Could you check a few things on this drawing? It's one solid part, dimensions in mm from its lowest x, y, z. A direction names the side the tool comes from. Give positions to 0.01 mm unless a question says otherwise; leave off trailing zeros. Order: outer loops, then holes, each group sorted by start corner. A loop starts at its lowest first (then second) coordinate and runs counter-clockwise, first axis right, second up. Notation, with made-up numbers: (-11.75, 75) - (29.25, 75) arc R15 cw to (29.25, 89) - close; hole circle Ø10 at (-12.5, 29.5). An arc over 180 degrees is marked (long way). Put each result on its own line as item: value.
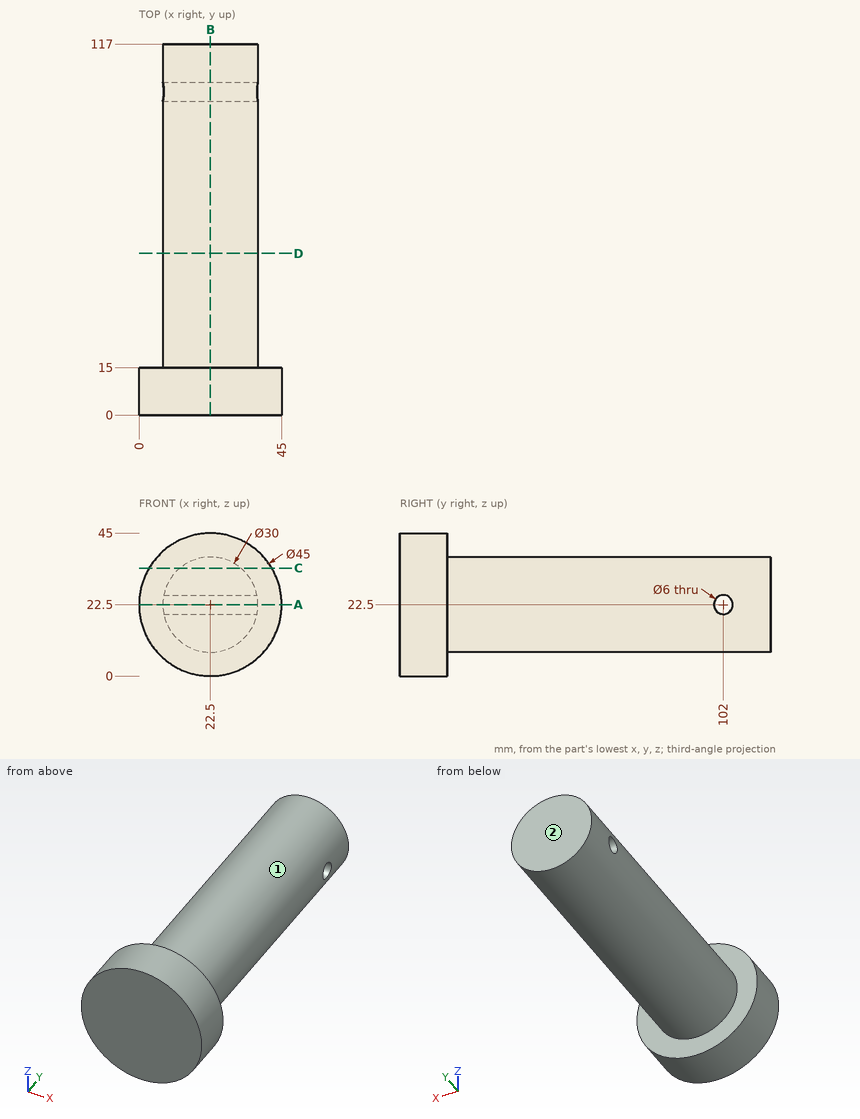
1) Suppose I cut it at D-D, the plane y = 51. List the corners of the cut face in (x, z) for me, and give its area (3 significant figures).
Filled in:
outline: circle Ø30 at (22.5, 22.5)
area: 707 mm^2
2) Which directions (+Z, -Z, +X, -X, +Y, -Y) give clear straight access to the entire face, cutting with the end or side of a thin tool? Please do the marked faces 1 and 2.
Filled in:
face 1: +Y
face 2: +Z, -Z, +X, -X, +Y
3) Suppose I cut it at B-B, the plane x = 22.5. List the corners of the cut face in (y, z) for me.
Filled in:
outline: (0, 0) - (15, 0) - (15, 7.5) - (117, 7.5) - (117, 37.5) - (15, 37.5) - (15, 45) - (0, 45) - close; hole circle Ø6 at (102, 22.5)
4) I'm going to push flat-ended pins straight in: pin 1 (8 mm diameter, centred on x = 9, y = 84.5, fed in from -Z); pin 2 (1.5 mm diameter, centred on y = 17, z = 28.5, fed in from +X); pin 3 (5 mm diameter, centred on y = 35.5, z = 37.5, fed in from +X). Where does each tip first touch, or does it pass through?
Filled in:
pin 1: stops at z = 10.89
pin 2: stops at x = 36.55
pin 3: stops at x = 30.79
5) Suppose I cut it at C-C, the plane z = 34. List the corners of the cut face in (x, y) for me, and give its area (3 significant figures).
Filled in:
outline: (3.16, 0) - (41.84, 0) - (41.84, 15) - (32.13, 15) - (32.13, 117) - (12.87, 117) - (12.87, 15) - (3.16, 15) - close
area: 2,540 mm^2
6) Suppose I cut it at A-A, the plane z = 22.5. List the corners of the cut face in (x, y) for me, and give its area (4 significant figures).
Filled in:
outline: (0, 0) - (45, 0) - (45, 15) - (37.5, 15) - (37.5, 99) - (7.5, 99) - (7.5, 15) - (0, 15) - close; (7.5, 105) - (37.5, 105) - (37.5, 117) - (7.5, 117) - close
area: 3,555 mm^2
7) If I drill on line 1 (Y direction, x = 26, z = 22.5); line 2 (Y direction, x = 19, z = 23.5); line 3 (Z direction, x = 29, y = 102), over which ranges is the centre line in solid material (lowest first)? Write a range as [from, to].
Filled in:
line 1: y = [0, 99], [105, 117]
line 2: y = [0, 99.17], [104.83, 117]
line 3: z = [8.98, 19.5], [25.5, 36.02]
